Check sheet for the modelled part. Datum: model origin and axes. Units: mm. A direction names the side the tool comes from. Give positions to 0.01 mm unless a question says otherwise; leave off trailing zeros.
```python
from build123d import *

# Parameters (mm, degrees)
SKETCH_1_W             = 23.5
SKETCH_1_H             = 12
EXTRUDE_1_DEPTH        = 75
HOLE_WIZARD_M6_1_D     = 5
HOLE_WIZARD_M6_1_DEPTH = 19
HOLE_WIZARD_M6_1_TIP   = 1.502151548
HOLE_WIZARD_M6_2_D     = 5
HOLE_WIZARD_M6_2_DEPTH = 19
HOLE_WIZARD_M6_2_TIP   = 1.502151548


with BuildPart() as part:
    # 草图1 → 凸台-拉伸1 (new, symmetric)
    with BuildSketch(Plane(origin=(0, 0, 0), x_dir=(0, 0, -1), z_dir=(1, 0, 0))):
        Polygon((-15, 15), (-11.5, 15), (-11.5, 13.5), (-11, 13.5), (-11, 12), (-9.5, 12), (-9.5, 15), (-8, 15), (-8, 12.5), (-5, 12.5), (-5, 15), (5, 15), (5, 12.5), (8, 12.5), (8, 15), (9.5, 15), (9.5, 12), (11, 12), (11, 13.5), (11.5, 13.5), (11.5, 15), (15, 15), (15, 8), (12.5, 8), (12.5, 5), (15, 5), (15, -5), (12.5, -5), (12.5, -8), (15, -8), (15, -15), (11.5, -15), (11.5, -13.5), (11, -13.5), (11, -12), (9.5, -12), (9.5, -15), (8, -15), (8, -12.5), (5, -12.5), (5, -15), (-5, -15), (-5, -12.5), (-8, -12.5), (-8, -15), (-9.5, -15), (-9.5, -12), (-11, -12), (-11, -13.5), (-11.5, -13.5), (-11.5, -15), (-15, -15), align=None)
        with BuildLine():
            Line((12, -10.5), (12, -8.5))
            ThreePointArc((12, -8.5), (11.853553391, -8.146446609), (11.5, -8))
            Line((11.5, -8), (-11.5, -8))
            ThreePointArc((-11.5, -8), (-11.853553391, -8.146446609), (-12, -8.5))
            Line((-12, -8.5), (-12, -10.5))
            ThreePointArc((-12, -10.5), (-11.853553391, -10.853553391), (-11.5, -11))
            Line((-11.5, -11), (11.5, -11))
            ThreePointArc((11.5, -11), (11.853553391, -10.853553391), (12, -10.5))
        make_face(mode=Mode.SUBTRACT)
        with BuildLine():
            Line((-11.5, 11), (11.5, 11))
            ThreePointArc((11.5, 11), (11.853553391, 10.853553391), (12, 10.5))
            Line((12, 10.5), (12, 8.5))
            ThreePointArc((12, 8.5), (11.853553391, 8.146446609), (11.5, 8))
            Line((11.5, 8), (-11.5, 8))
            ThreePointArc((-11.5, 8), (-11.853553391, 8.146446609), (-12, 8.5))
            Line((-12, 8.5), (-12, 10.5))
            ThreePointArc((-12, 10.5), (-11.853553391, 10.853553391), (-11.5, 11))
        make_face(mode=Mode.SUBTRACT)
        Rectangle(SKETCH_1_W, SKETCH_1_H, mode=Mode.SUBTRACT)
    extrude(amount=EXTRUDE_1_DEPTH, both=True)

    # M6 螺纹孔1
    with Locations(Plane(origin=(0, -15, 0), x_dir=(-1, 0, 0), z_dir=(0, -1, 0))):
        with Locations((-55, 0), (-40, 0), (55, 0), (40, 0)):
            Hole(HOLE_WIZARD_M6_1_D / 2, depth=HOLE_WIZARD_M6_1_DEPTH)
            with Locations((0, 0, -(HOLE_WIZARD_M6_1_DEPTH + HOLE_WIZARD_M6_1_TIP / 2))):  # 118° drill point
                Cone(0, HOLE_WIZARD_M6_1_D / 2, HOLE_WIZARD_M6_1_TIP, mode=Mode.SUBTRACT)

    # M6 螺纹孔2
    with Locations(Plane(origin=(0, 0, -15), x_dir=(-1, 0, 0), z_dir=(0, 0, -1))):
        with Locations((-55, 0), (-40, 0), (40, 0), (55, 0), (-4, 0), (4, 0)):
            Hole(HOLE_WIZARD_M6_2_D / 2, depth=HOLE_WIZARD_M6_2_DEPTH)
            with Locations((0, 0, -(HOLE_WIZARD_M6_2_DEPTH + HOLE_WIZARD_M6_2_TIP / 2))):  # 118° drill point
                Cone(0, HOLE_WIZARD_M6_2_D / 2, HOLE_WIZARD_M6_2_TIP, mode=Mode.SUBTRACT)


solid = part.part
```
(1) Release check for a two-part mould opening along Y. For faces 1 (the face through (1, -13, -9.5)), 2 (the face through (42.31, -0.96, -13.35)), 3 (the face through (1, 15, 0)), 4 (the face through (1, 0, -11.75)) record: released by +Y, released by -Y, zero draft, split by the parting line, or undercut.
(2) Thickness scan on L1, parallel to Y at x = 67.5, z = 6.5; L2, parallel to Y at x = -34.5, z = 3.75; L3, parallel to Z at x = -40, y = -13.4. Record the ranges inside material, lowest first.
(3) Tool access check on faces 5 (the face through (-37.69, -0.96, -13.35)), 6 (the face through (1, 8, -14)), 7 (the face through (1, 11, 0)), 8 (the face through (1, 12.5, 7)). Record the directions out of +Z, -Z, +X, -X, +Y, -Y that give a thin tool (end or side, any length) a straight path to the whole face; none if there is none.
(4) Sectioned sample at A-A (y = 0). Count the separate pieces of the cut face and the enclosed holes in it, plus the area to 4 significant figures.
(5) Go/stop test with flat-tipped pins: P1, Ø3, axis at x = -40, z = 0, coming from the -Y side; P2, Ø1.5, axis at x = 50, z = 5.5, coming from the +Y side; P3, Ø1, axis at x = 11, y = -6, coming from the -Z side. Record where each tip stops, or that it passes through.
Values follow:
1. face 1: zero draft
1. face 2: undercut
1. face 3: released by +Y
1. face 4: undercut
2. L1: y = -12.5 to -11, -8 to -6, 6 to 8, 11 to 12.5
2. L2: y = -15 to -11, -8 to -6, 6 to 8, 11 to 15
2. L3: z = -15 to -11, -9.5 to -8, -5 to -2.5, 2.5 to 5, 8 to 9.5, 11 to 15
3. face 5: -Z
3. face 6: -Z, +X, -X
3. face 7: +X, -X
3. face 8: +X, -X, +Y
4. separate pieces: 8
4. enclosed holes: 0
4. area: 877.5 mm2
5. P1: stops at y = 6
5. P2: stops at y = 15
5. P3: stops at z = -12.5
